from build123d import *

# Parameters (mm, degrees)
F0_W     = 64.0207
F0_H     = 124.1298
F1_DEPTH = 5.9182
F2_R     = 2.1336
F3_DEPTH = 5.9192
F4_SIZE  = 3.429
F6_DEPTH = 22.86


with BuildPart() as f1:
    # F0 (on Front) → F1 (new body)
    with BuildSketch(Plane.XZ):
        Rectangle(F0_W, F0_H)
    extrude(amount=F1_DEPTH)

    # F2 (on face) → F3 (cut, through all)
    with BuildSketch(Plane(origin=(0, 0, 0), x_dir=(-1, 0, 0), z_dir=(0, 1, 0))):
        with Locations((-25.72385, 51.2953)):
            Circle(F2_R)
        with Locations((25.72385, 51.2953)):
            Circle(F2_R)
        with Locations((25.72385, -51.2953)):
            Circle(F2_R)
        with Locations((-25.72385, -51.2953)):
            Circle(F2_R)
    extrude(amount=-F3_DEPTH, mode=Mode.SUBTRACT)

    # F4
    f4_edges = [f1.edges().sort_by_distance(p)[0] for p in [
        (0, -5.9182, 62.0649),
        (-32.01035, -5.9182, 0),
        (0, -5.9182, -62.0649),
        (32.01035, -5.9182, 0),
    ]]
    chamfer(f4_edges, length=F4_SIZE)

    # F5 (on Right) → F6 (join, symmetric)
    with BuildSketch(Plane.YZ):
        Polygon((11.1125, 52.6669), (0, 52.6669), (0, -55.790792), (65.0875, -41.327979), (65.0875, -73.077979), (106.3625, -73.077979), (106.3625, 22.172021), align=None)
    extrude(amount=F6_DEPTH, both=True)


solid = f1.part
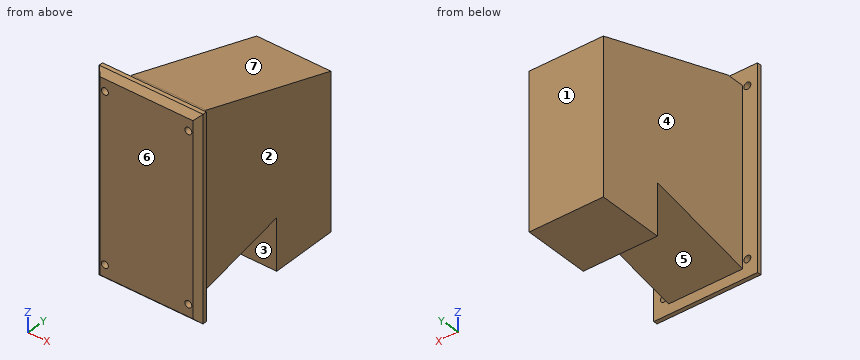
Source: CAD feature listing. Evaluate the final solid. Frame: model axes, mm. Face numbers are marked on the shaded views. A direction names the side the tool comes from. Coordinates: 2 decimals unless noted, no trailing zeros. Loops run counter-clockwise (first coordinate to the right, second up) from the corner with the lowest first, then second, coordinate; pieces in that order, holes last. Notation, with made-up numbers: M 82.5,75 L 141.5,75 A14 ccw 141.5,92 Z; hole C 45,-21.5 d5. An arc over 180 degrees is marked long. Answer in a Markdown table with one row per item.
Q1. Set-up query: the marked faces 1, 2, 3 and 4. Return all of +Z, -Z, +X, -X, +Y, -Y with unobstructed straight access to the full face (end or side cutting, diameter ignored); none if empty.
Answers below:
| item | result |
|---|---|
| face 1 | +Z, -Z, +X, -X, +Y |
| face 2 | +Z, -Z, +X, +Y |
| face 3 | -Z, +X, -X |
| face 4 | +Z, -Z, -X, +Y |
Q2. Section B-B on x = -26. Return the cut outline in (y, z), plus the area to 3 significant figures.
Answers below:
| item | result |
|---|---|
| outline | M -5.92,-58.64 L -2.49,-62.06 L 0,-62.06 L 0,-53.41 L -5.92,-53.41 Z; M -5.92,-49.18 L 0,-49.18 L 0,49.18 L -5.92,49.18 Z; M -5.92,53.41 L 0,53.41 L 0,62.06 L -2.49,62.06 L -5.92,58.64 Z |
| area | 673 mm^2 |
Q3. Draft query along Y for the marked faces 5, 6 and 7. Return one class per face: pulls with the +Y half, pulls with the -Y half, needs draft (parallel to the pull), parting line crosses it, or undercut.
Answers below:
| item | result |
|---|---|
| face 5 | undercut |
| face 6 | pulls with the -Y half |
| face 7 | pulls with the +Y half |
Q4. Section C-C on x = -16.5. Return the cut outline in (y, z), plus the area to 3 significant figures.
Answers below:
| item | result |
|---|---|
| outline | M -5.92,-58.64 L -2.49,-62.06 L 0,-62.06 L 0,-55.79 L 65.09,-41.33 L 65.09,-73.08 L 106.36,-73.08 L 106.36,22.17 L 11.11,52.67 L 0,52.67 L 0,62.06 L -2.49,62.06 L -5.92,58.64 Z |
| area | 11,000 mm^2 |
Q5. First-contact query: pin 1 (9 mm diameter, centred on x = 8.5, y = 7, fed in from +Z); pin 2 (5.5 mm diameter, centred on x = 25.72, z = -51.3, fed in from +Y); pin 3 (12 mm diameter, centred on x = -17, y = 39, fed in from -Z); pin 4 (2 mm diameter, centred on x = 24.5, y = 79.5, fed in from +Z). Flat tips, straight axial feed; report the tip coordinate or a pass-through.
Answers below:
| item | result |
|---|---|
| pin 1 | stops at z = 52.67 |
| pin 2 | stops at y = 0 |
| pin 3 | stops at z = -48.46 |
| pin 4 | passes through |
Q6. Ray query, probe 1 along X at (y, z) = (62, -29); probe 2 along Y at (x, z) = (-7.5, -66); probe 3 along Y at (x, z) = (-26, -32). Return the intervals inside material, ascending. Write a range as from..to.
Answers below:
| item | result |
|---|---|
| probe 1 | x = -22.86..22.86 |
| probe 2 | y = 65.09..106.36 |
| probe 3 | y = -5.92..0 |
Q7. Section A-A on z = -22. Return the cut outline in (x, y).
Answers below:
| item | result |
|---|---|
| outline | M -32.01,-2.49 L -28.58,-5.92 L 28.58,-5.92 L 32.01,-2.49 L 32.01,0 L 22.86,0 L 22.86,106.36 L -22.86,106.36 L -22.86,0 L -32.01,0 Z |
Q8. Section D-D on z = 43. Return the cut outline in (x, y), plus the area to 3 significant figures.
Answers below:
| item | result |
|---|---|
| outline | M -32.01,-2.49 L -28.58,-5.92 L 28.58,-5.92 L 32.01,-2.49 L 32.01,0 L 22.86,0 L 22.86,41.31 L -22.86,41.31 L -22.86,0 L -32.01,0 Z |
| area | 2,260 mm^2 |
